Check sheet for the modelled part. Datum: model origin and axes. Units: mm. Coordinates: 2 decimals unless noted, no trailing zeros. Order: outer loops, then holes, each group sorted by start corner. A loop starts at its lowest first (then second) coordinate and runs counter-clockwise, first axis right, second up.
1. Gauge pin test, flat ends, axial feed: pin 1 Ø0.9 at (x, z) = (-16, -15) entering from +Y; pin 2 Ø10 at (y, z) = (19, 7) entering from +X; pin 3 Ø8 at (y, z) = (270.5, 6) entering from -X. Record the tip position at first contact, or that the pin passes through.
2. Thickness scan on line 1 (Z direction, x = -15.5, y = 36.95); line 2 (Z direction, x = 0, y = 39.8). Record the ranges inside material, lowest first.
3. Cross-section at C-C (y = 76). Enter the section's corners in (x, z).
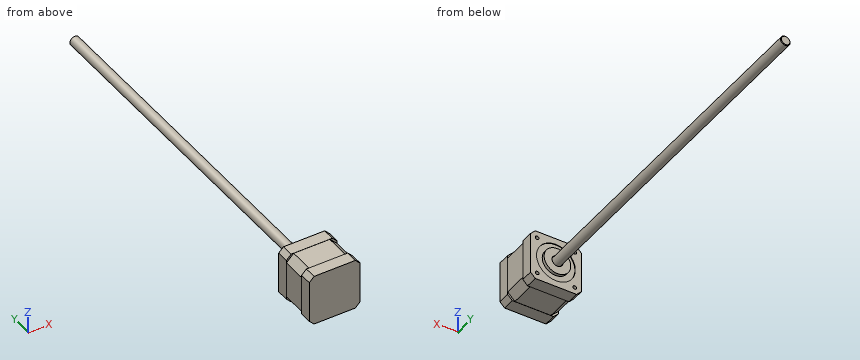
Autodesk Inventor part; units mm, degrees
ref_plane "Work Plane1" through (0, 20, 0) normal (0, 1, 0) x (1, 0, 0)
ref_plane "YZ Plane" through (0, 0, 0) normal (1, 0, 0) x (0, 1, 0)
ref_plane "XZ Plane" through (0, 0, 0) normal (0, 1, 0) x (-1, 0, 0)
sketch "Sketch1" plane through (0, 0, 0) normal (0, 1, 0) x (-1, 0, 0)
  line L0 (-21, 21) -> (21, 21)
  line L1 (21, 21) -> (21, -21)
  line L2 (21, -21) -> (-21, -21)
  line L3 (-21, -21) -> (-21, 21)
  line L4 (-21, 21) -> (21, -21) construction
  line L5 (21, 21) -> (-21, -21) construction
  point P0 (0, 0)
  dimension "d0" = 42
  dimension "d1" = 42
extrude "Extrusion1" add sketch "Sketch1" along normal blind 40
ref_plane "Work Plane1" through (0, 20, 0) normal (0, 1, 0) x (1, 0, 0)
sketch "Sketch2" plane through (0, 40, 0) normal (0, 1, 0) x (1, 0, 0)
  line L0 (0, -38.0423) -> (-38.0423, 0)
  line L1 (-38.0423, 0) -> (0, 38.0423)
  line L2 (0, 38.0423) -> (38.0423, 0)
  line L3 (38.0423, 0) -> (0, -38.0423)
  line L4 (0, -38.0423) -> (0, 38.0423) construction
  line L5 (-38.0423, 0) -> (38.0423, 0) construction
  line L6 (-21, 21) -> (-21, -21)
  circle A0 centre (0, 0) radius 250
  dimension "d4" = 53.8
  dimension "d5" = 53.8
  dimension "d6" = 500
extrude "Extrusion2" cut sketch "Sketch2" against normal blind 10
sketch "Sketch3" plane through (0, 20, 0) normal (0, 1, 0) x (1, 0, 0)
  line L0 (-20.9, -20.9) -> (20.9, -20.9)
  line L1 (20.9, -20.9) -> (20.9, 20.9)
  line L2 (20.9, 20.9) -> (-20.9, 20.9)
  line L3 (-20.9, 20.9) -> (-20.9, -20.9)
  line L4 (-21, -21) -> (-21, -17.0423)
  line L5 (21, -21) -> (17.0423, -21)
  line L6 (21, 21) -> (21, 17.0423)
  line L7 (-21, 21) -> (-17.0423, 21)
  circle A0 centre (0, 0) radius 200
  dimension "d9" = 0.1
  dimension "d10" = 0.1
  dimension "d11" = 0.1
  dimension "d12" = 0.1
  dimension "d13" = 400
extrude "Extrusion3" cut sketch "Sketch3" along normal up to surface (10 mm away)
chamfer "Chamfer1" distance 6 angle 45 4 edges at (20.9, 25, 20.9) (20.9, 25, -20.9) (-20.9, 25, 20.9) (-20.9, 25, -20.9)
mirror "Mirror1" about plane through (0, 20, 0) normal (0, 1, 0) of "Extrusion3", "Extrusion2", "Chamfer1"
sketch "Sketch4" plane through (0, 40, 0) normal (0, 1, 0) x (1, 0, 0)
  circle A0 centre (0, 0) radius 11
  dimension "d19" = 22
extrude "Extrusion4" add sketch "Sketch4" along normal blind 2
sketch "Sketch5" plane through (0, 40, 0) normal (0, 1, 0) x (1, 0, 0)
  circle A0 centre (0, 0) radius 11
  line L0 (17.0423, -21) -> (21, -17.0423)
  line L1 (21, -17.0423) -> (21, 17.0423)
  line L2 (21, 17.0423) -> (17.0423, 21)
  line L3 (17.0423, 21) -> (-17.0423, 21)
  line L4 (-17.0423, 21) -> (-21, 17.0423)
  line L5 (-21, 17.0423) -> (-21, -17.0423)
  line L6 (-21, -17.0423) -> (-17.0423, -21)
  line L7 (-17.0423, -21) -> (17.0423, -21)
  circle A1 centre (0, 0) radius 16
  dimension "d22" = 32
extrude "Extrusion5" cut sketch "Sketch5" against normal blind 0.5 contours A1
sketch "Sketch6" plane through (0, 42, 0) normal (0, 1, 0) x (1, 0, 0)
  circle A0 centre (0, 0) radius 4.5
  dimension "d25" = 9
extrude "Extrusion6" cut sketch "Sketch6" against normal blind 2
sketch "Sketch7" plane through (0, 40, 0) normal (0, 1, 0) x (1, 0, 0)
  circle A0 centre (0, 0) radius 4
  dimension "d28" = 8
extrude "Extrusion7" add sketch "Sketch7" along normal blind 300
thread "Thread1"
chamfer "Chamfer2" distance 0.5 angle 45 1 edges at (-4, 340, 0)
sketch "Sketch8" plane through (0, 40, 0) normal (0, 1, 0) x (1, 0, 0)
  circle A0 centre (0, 0) radius 16 construction
  line L0 (17.0423, -21) -> (21, -17.0423) construction
  line L1 (21, -17.0423) -> (21, 17.0423) construction
  line L2 (21, 17.0423) -> (17.0423, 21) construction
  line L3 (17.0423, 21) -> (-17.0423, 21) construction
  line L4 (-17.0423, 21) -> (-21, 17.0423) construction
  line L5 (-21, 17.0423) -> (-21, -17.0423) construction
  line L6 (-21, -17.0423) -> (-17.0423, -21) construction
  line L7 (-17.0423, -21) -> (17.0423, -21) construction
  line L8 (-15.5, -15.5) -> (15.5, -15.5) construction
  line L9 (15.5, -15.5) -> (15.5, 15.5) construction
  line L10 (15.5, 15.5) -> (-15.5, 15.5) construction
  line L11 (-15.5, 15.5) -> (-15.5, -15.5) construction
  line L12 (-15.5, -15.5) -> (15.5, 15.5) construction
  line L13 (15.5, -15.5) -> (-15.5, 15.5) construction
  circle A1 centre (-15.5, 15.5) radius 1.5
  circle A2 centre (15.5, 15.5) radius 1.5
  circle A3 centre (15.5, -15.5) radius 1.5
  circle A4 centre (-15.5, -15.5) radius 1.5
  dimension "d36" = 31
  dimension "d37" = 31
  dimension "d38" = 3
  dimension "d39" = 3
  dimension "d40" = 3
  dimension "d41" = 3
extrude "Extrusion8" cut sketch "Sketch8" against normal blind 5
thread "Thread2"
pattern_circular "Circular Pattern1" count 4 over 360 about axis through (0, 40, 0) along (0, 1, 0) of "Extrusion8"
equation "\"d9\" = d10"
equation "\"d11\" = d10"
equation "\"d12\" = d10"
properties part number "linear_stepper_350mm"
Data:
1. pin 1: stops at y = 35
1. pin 2: stops at x = 20.9
1. pin 3: stops at x = -3.46
2. line 1: z = -21 to -17, -14 to 14, 17 to 21
2. line 2: z = -21 to -16, -11 to 11, 16 to 21
3. outline: circle Ø8 at (0, 0)
